from build123d import *

# Parameters (mm, degrees)
SKETCH2_R           = 3.175
SKETCH2_R_2         = 2
SKETCH2_R_3         = 1.905
SKETCH2_R_4         = 1.999999991
BOSS_EXTRUDE1_DEPTH = 6.35
FILLET2_R           = 2.54
FILLET3_R           = 2.54
FILLET4_R           = 2.54
FILLET5_R           = 2.54


with BuildPart() as part:
    # Sketch2 → Boss-Extrude1 (new body)
    with BuildSketch(Plane(origin=(0, 0, 0), x_dir=(1, 0, 0), z_dir=(0, 1, 0))):
        with BuildLine():
            Line((13.846627418, -27.11715969), (17.295902343, -28.359470371))
            Line((17.295902343, -28.359470371), (17.295902343, -164.950770806))
            Line((17.295902343, -164.950770806), (-5.788689103, -224.106088723))
            Line((-5.788689103, -224.106088723), (-16.51, -231.775))
            Line((-16.51, -231.775), (-16.51, -190.41700733))
            Line((-16.51, -190.41700733), (-8.721771923, -190.41700733))
            Line((-8.721771923, -190.41700733), (-16.51, -118.11))
            Line((-16.51, -118.11), (-16.51, -40.527182032))
            Line((-16.51, -40.527182032), (-12.5603, 0))
            ThreePointArc((-12.5603, 0), (0, 12.5603), (12.5603, 0))
            Line((12.5603, 0), (11.834308479, -23.392641285))
            ThreePointArc((11.834308479, -23.392641285), (12.129138804, -25.639224299), (13.846627418, -27.11715969))
        make_face()
        with Locations(Location((0, 0, 0), (0, 0, 270))):
            Circle(SKETCH2_R, mode=Mode.SUBTRACT)
        with Locations(Location((-11.43, -219.075, 0), (0, 0, 270))):
            Circle(SKETCH2_R_2, mode=Mode.SUBTRACT)
        with Locations(Location((-11.43, -212.725, 0), (0, 0, 270))):
            Circle(SKETCH2_R_2, mode=Mode.SUBTRACT)
        with Locations(Location((-11.43, -206.375, 0), (0, 0, 270))):
            Circle(SKETCH2_R_2, mode=Mode.SUBTRACT)
        with Locations(Location((-11.43, -200.025, 0), (0, 0, 270))):
            Circle(SKETCH2_R_2, mode=Mode.SUBTRACT)
        with Locations(Location((-10.6553, -63.5, 0), (0, 0, 270))):
            Circle(SKETCH2_R_3, mode=Mode.SUBTRACT)
        with Locations(Location((13.485902343, -38.1, 0), (0, 0, 270))):
            Circle(SKETCH2_R_4, mode=Mode.SUBTRACT)
        Polygon((-3.088444979, -200.025), (-8.437091633, -150.367410486), (11.707902343, -162.914359455), align=None, mode=Mode.SUBTRACT)
        Polygon((5.669829362, -152.570430441), (11.707902343, -156.331136136), (11.707902343, -148.173239335), align=None, mode=Mode.SUBTRACT)
        Polygon((-9.197164207, -143.310789567), (1.48362655, -149.963128939), (11.707902343, -142.517360277), (11.707902343, -83.82613362), (-6.752611098, -71.345410911), (-11.894481361, -75.089947663), (-11.894481361, -118.268516882), align=None, mode=Mode.SUBTRACT)
        with BuildLine():
            Line((-5.45038708, -57.047318199), (5.477174601, -46.119756518))
            Line((5.477174601, -46.119756518), (9.770631453, -46.119756518))
            Line((9.770631453, -46.119756518), (11.707902343, -77.037423395))
            Line((11.707902343, -77.037423395), (-4.240626345, -66.254995008))
            ThreePointArc((-4.240626345, -66.254995008), (-4.111536449, -61.554723114), (-5.45038708, -57.047318199))
        make_face(mode=Mode.SUBTRACT)
        Polygon((-5.48107582, -40.527182032), (-10.6553, -40.527182032), (-8.00152211, -13.297230483), (5.477174601, -13.297230483), (5.477174601, -31.974105906), (1.94113758, -40.527182032), align=None, mode=Mode.SUBTRACT)
        Polygon((-10.6553, -44.022777243), (-10.6553, -51.472145687), (-0.991335505, -44.022777243), align=None, mode=Mode.SUBTRACT)
    extrude(amount=BOSS_EXTRUDE1_DEPTH)

    # Fillet2
    fillet2_edges = [part.edges().sort_by_distance(p)[0] for p in [
        (-8.721771923, 3.175, 190.41700733),
    ]]
    fillet(fillet2_edges, radius=FILLET2_R)

    # Fillet3
    fillet3_edges = [part.edges().sort_by_distance(p)[0] for p in [
        (-5.788689103, 3.175, 224.106088723),
    ]]
    fillet(fillet3_edges, radius=FILLET3_R)

    # Fillet4
    fillet4_edges = [part.edges().sort_by_distance(p)[0] for p in [
        (-16.51, 3.175, 231.775),
    ]]
    fillet(fillet4_edges, radius=FILLET4_R)

    # Fillet5
    fillet5_edges = [part.edges().sort_by_distance(p)[0] for p in [
        (17.295902343, 3.175, 164.950770806),
    ]]
    fillet(fillet5_edges, radius=FILLET5_R)


solid = part.part
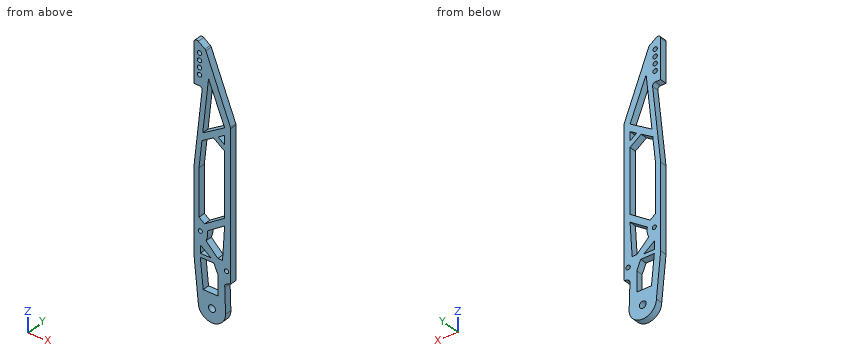
The model under review builds one solid part; all positions refer to its coordinate system, in mm. Give positions to 0.01 mm unless a question says otherwise; leave off trailing zeros. Order: outer loops, then holes, each group sorted by start corner. A loop starts at its lowest first (then second) coordinate and runs counter-clockwise, first axis right, second up. Notation, with made-up numbers: (-9.5, -8) -> (49.5, -8) arc R17 cw to (49.5, 2) -> close; hole circle Ø2 at (35, 63.25). An arc over 180 degrees is marked (long way). Write item = value, one per line. Start each with the question number.
(1) For L1, parallel to X at y = 4.25, z = 0 (3 decimals); L2, parallel to X at y = 4.25, z = 51; L3, parallel to X at y = 3, z = 112.5, list the stretches that pass through material, from the lowest coordinate up. Write a range as from..to.
(2) For pin 1 Ø1.9 at (x, y) = (-7.5, 2) entering from -Z; pin 2 Ø3 at (x, y) = (-7.5, 1.5) entering from +Z; pin 3 Ø1.9 at (y, z) = (3.5, 22.5) entering from -X, all flat-tipped, find the tip position at first contact; note any pin that passes through.
(3) Take a section at A-A (z = 38.1). Write out the cut boundary in (x, y).
(4) Take a section at B-B (y = 1). State how many separate pieces and enclosed holes the cut face has, plus the area to 3 significant figures.
Returned:
q1.L1 = -12.56..-3.175, 3.175..12.56
q1.L2 = -16.51..-10.66, -10.04..0.6, 10.08..17.3
q1.L3 = -16.51..-11.89, 11.71..17.3
q2.pin_1 = -10.72
q2.pin_2 = 226.4
q2.pin_3 = -14.85
q3.outline = (-16.27, 0) -> (-10.42, 0) -> (-10.42, 6.35) -> (-16.27, 6.35) -> close; (2.94, 0) -> (11.49, 0) -> (11.49, 6.35) -> (2.94, 6.35) -> close; (15.49, 0) -> (17.3, 0) -> (17.3, 6.35) -> (15.49, 6.35) -> close
q4.separate_pieces = 1
q4.enclosed_holes = 13
q4.area = 3,720 mm²
